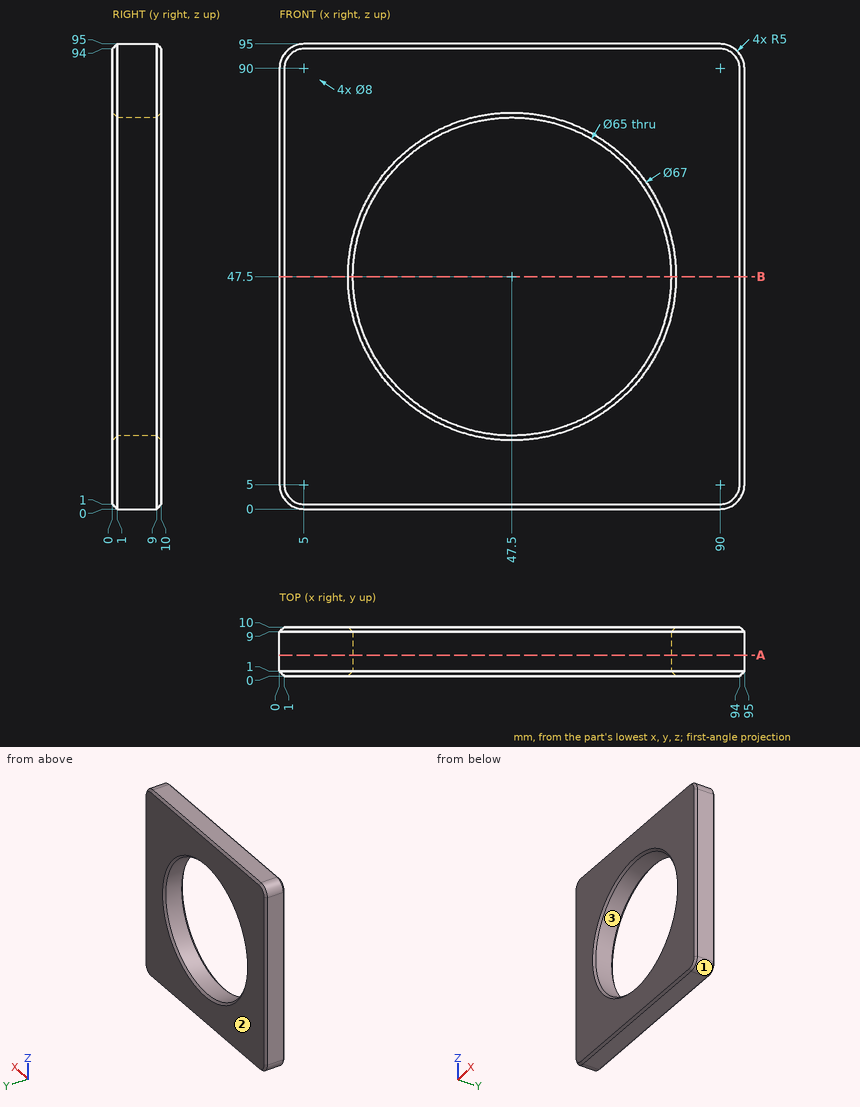
Input: dimensioned drawing with shaded views. Units: mm. Origin: part minimum x, y, z. Round coordinates to 2 decimals unless told otherwise and drop trailing zeros. Order: outer loops, then holes, each group sorted by start corner. A loop starts at its lowest first (then second) coordinate and runs counter-clockwise, first axis right, second up. Notation, with made-up numbers: (9.25, 32.25) - (60.25, 32.25) arc R28 ccw to (60.25, 50.25) - close; hole circle Ø7 at (23, -21). An arc over 180 degrees is marked (long way). Answer as a JSON object with one key per item and string values. Group by question number.
(1) Cut plane A-A (y = 4.25). Return loops of the section in (x, z).
(2) Draft query along Z for the marked faces 1, 2 and 3. Return one class per face: released by +Z, released by -Z, zero draft, split by the parting line, or undercut.
(3) Cut plane B-B (z = 47.5). Return loops of the section in (x, y), then the cut area to 3 significant figures.
(4) Material intervals for probe 1 along X at (y, z) = (4.5, 47.5); probe 2 along X at (y, z) = (1.5, 27.5); probe 3 along Z at (x, y) = (67.5, 9.5), sorted ascending. Write a range as from..to.
Here are the results:
{
 "1": {"outline": "(0, 5) arc R5 ccw to (5, 0) - (90, 0) arc R5 ccw to (95, 5) - (95, 90) arc R5 ccw to (90, 95) - (5, 95) arc R5 ccw to (0, 90) - close; hole circle Ø65 at (47.5, 47.5)"},
 "2": {"face 1": "released by -Z", "face 2": "zero draft", "face 3": "undercut"},
 "3": {"outline": "(0, 1) - (1, 0) - (14, 0) - (15, 1) - (15, 9) - (14, 10) - (1, 10) - (0, 9) - close; (80, 1) - (81, 0) - (94, 0) - (95, 1) - (95, 9) - (94, 10) - (81, 10) - (80, 9) - close", "area": "296 mm^2"},
 "4": {"probe 1": "x = 0..15, 80..95", "probe 2": "x = 0..21.88, 73.12..95", "probe 3": "z = 0.5..21.25, 73.75..94.5"}
}
